Geometry: see drawing. Coordinates: mm, zero at the bounding-box minimum. A direction names the side the tool comes from. Give positions to 0.01 mm unless a question says otherwise; leave off trailing zeros. Loops run counter-clockwise (first coordinate to the right, second up) from the corner with the lowest first, then second, coordinate; pieces in that order, holes last. Notation, with made-up numbers: (5, 26) -> (64, 26) arc R15 ccw to (64, 51) -> close; hole circle Ø2 at (-13.75, -10.5). An arc over 180 degrees is marked (long way). One line per question, with ' | ' between items.
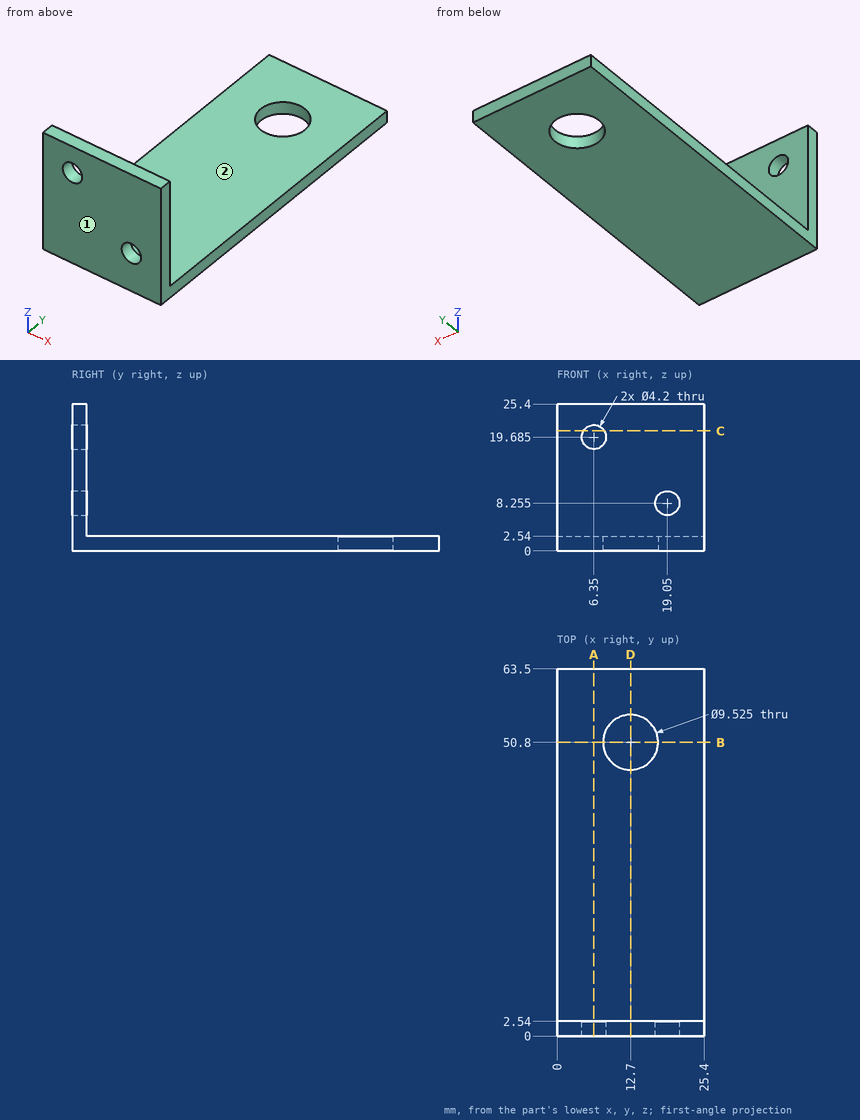
1. Section query B-B (y = 50.8). Output: boundary loops of the cut face in (x, z), then the cut area to 3 significant figures.
Determined:
outline: (0, 0) -> (7.94, 0) -> (7.94, 2.54) -> (0, 2.54) -> close; (17.46, 0) -> (25.4, 0) -> (25.4, 2.54) -> (17.46, 2.54) -> close | area: 40.3 mm2
2. Reachability of the marked faces 1 and 2 from +Z, -Z, +X, -X, +Y, -Y: full face, straight path, thin tool, end or side. Return the list, or none.
Determined:
face 1: +Z, -Z, +X, -X, -Y | face 2: +Z, +X, -X, +Y
3. Section query A-A (x = 6.35). Output: boundary loops of the cut face in (y, z) (3 decimals).
Determined:
outline: (0, 0) -> (63.5, 0) -> (63.5, 2.54) -> (2.54, 2.54) -> (2.54, 17.585) -> (0, 17.585) -> close; (0, 21.785) -> (2.54, 21.785) -> (2.54, 25.4) -> (0, 25.4) -> close
4. Section query C-C (z = 20.75). Output: boundary loops of the cut face in (x, y).
Determined:
outline: (0, 0) -> (4.54, 0) -> (4.54, 2.54) -> (0, 2.54) -> close; (8.16, 0) -> (25.4, 0) -> (25.4, 2.54) -> (8.16, 2.54) -> close
5. Ray query, line 1 along Z through (x, y) = (6.35, 1.35) (3 decimals); line 2 along Z through (x, y) = (19.05, 1.4) (3 decimals); line 3 along Y through (x, z) = (12.7, 0.7). Return the intervals inside material, ascending. Write a range as from..to.
Determined:
line 1: z = 0..17.585, 21.785..25.4 | line 2: z = 0..6.155, 10.355..25.4 | line 3: y = 0..46.04, 55.56..63.5
6. Pin query (flat end, axial travel): P1, Ø8, axis at x = 17, z = 12, coming from the +Y side; P2, Ø10, axis at x = 16, y = 35, coming from the +Z side. Return the tip coordinate at first contact, or that it passes through.
Determined:
P1: stops at y = 2.54 | P2: stops at z = 2.54
7. Section query D-D (x = 12.7). Output: boundary loops of the cut face in (y, z).
Determined:
outline: (0, 0) -> (46.04, 0) -> (46.04, 2.54) -> (2.54, 2.54) -> (2.54, 25.4) -> (0, 25.4) -> close; (55.56, 0) -> (63.5, 0) -> (63.5, 2.54) -> (55.56, 2.54) -> close
